Input: part model. Units: mm. Frame: model coordinates. Coordinates: 2 decimals unless noted, no trailing zeros. Write each loop counter-clockwise with the first axis right and the second up, starting at its lowest first coordinate (ties: lowest second). Pieces come first, ordered by that corner, then holes. Notation, with made-up numbers: (47.5, 51.5) -> (106.5, 51.5) arc R7 ccw to (106.5, 63.5) -> close; hole circle Ø5 at (20.25, 31.5). An arc over 180 degrees is marked (long way). Use one line per item in the form item = value. Start each with the question number.
(1) Cut plane C-C on y = 14.5. Return the cut outline in (x, z).
(2) Cut plane B-B on z = 1056. Return the cut outline in (x, y), plus the area to 3 significant figures.
(3) Cut plane A-A on x = -239. Return the cut outline in (y, z).
(4) Ray query, line 1 along Z through (x, y) = (171.5, -68). Return the intervals inside material, ascending.
(5) Pull-direction query (Z, two-part tool) for faces 1 (the face through (-6, 3, 20)), 2 (the face through (-6, 3, 1220)), 3 (the face through (-6, 3, 900)), 4 (the face through (-35, -200, 607)); classes: released by +Z, released by -Z, zero draft, split by the parting line, or undercut.
```python
from build123d import *

# Parameters (mm, degrees)
F4_W      = 900
F4_H      = 400
F6_DEPTH  = 1220
F7_DEPTH  = 280
F11_DEPTH = 280
F12_DEPTH = 280
F13_DEPTH = 280


with BuildPart() as f6:
    # F4 (on Top) → F6 (new body)
    with BuildSketch(Plane.XY):
        Rectangle(F4_W, F4_H)
    extrude(amount=F6_DEPTH)

    # F5 (on offset) → F7 (cut)
    with BuildSketch(Plane.XY.offset(300)):
        Polygon((-430, 198), (-448, 198), (-448, 180), (-450, 180), (-450, -180), (-448, -180), (-448, -198), (-430, -198), (-430, -200), (430, -200), (430, -198), (448, -198), (448, -180), (450, -180), (450, 180), (448, 180), (448, 198), (430, 198), (430, 200), (-430, 200), align=None)
    extrude(amount=-F7_DEPTH, mode=Mode.SUBTRACT)

    # F8 (on offset) → F11 (cut)
    with BuildSketch(Plane.XY.offset(600)):
        Polygon((-430, 198), (-448, 198), (-448, 180), (-450, 180), (-450, -180), (-448, -180), (-448, -198), (-430, -198), (-430, -200), (430, -200), (430, -198), (448, -198), (448, -180), (450, -180), (450, 180), (448, 180), (448, 198), (430, 198), (430, 200), (-430, 200), align=None)
    extrude(amount=-F11_DEPTH, mode=Mode.SUBTRACT)

    # F9 (on offset) → F12 (cut)
    with BuildSketch(Plane.XY.offset(900)):
        Polygon((-430, 198), (-448, 198), (-448, 180), (-450, 180), (-450, -180), (-448, -180), (-448, -198), (-430, -198), (-430, -200), (430, -200), (430, -198), (448, -198), (448, -180), (450, -180), (450, 180), (448, 180), (448, 198), (430, 198), (430, 200), (-430, 200), align=None)
    extrude(amount=-F12_DEPTH, mode=Mode.SUBTRACT)

    # F10 (on offset) → F13 (cut)
    with BuildSketch(Plane.XY.offset(1200)):
        Polygon((-430, 198), (-448, 198), (-448, 180), (-450, 180), (-450, -180), (-448, -180), (-448, -198), (-430, -198), (-430, -200), (430, -200), (430, -198), (448, -198), (448, -180), (450, -180), (450, 180), (448, 180), (448, 198), (430, 198), (430, 200), (-430, 200), align=None)
    extrude(amount=-F13_DEPTH, mode=Mode.SUBTRACT)


solid = f6.part
```
Values:
q1.outline = (-450, 0) -> (450, 0) -> (450, 20) -> (-450, 20) -> close; (-450, 300) -> (450, 300) -> (450, 320) -> (-450, 320) -> close; (-450, 600) -> (450, 600) -> (450, 620) -> (-450, 620) -> close; (-450, 900) -> (450, 900) -> (450, 920) -> (-450, 920) -> close; (-450, 1200) -> (450, 1200) -> (450, 1220) -> (-450, 1220) -> close
q2.outline = (-450, -200) -> (-430, -200) -> (-430, -198) -> (-448, -198) -> (-448, -180) -> (-450, -180) -> close; (-450, 180) -> (-448, 180) -> (-448, 198) -> (-430, 198) -> (-430, 200) -> (-450, 200) -> close; (430, -200) -> (450, -200) -> (450, -180) -> (448, -180) -> (448, -198) -> (430, -198) -> close; (430, 198) -> (448, 198) -> (448, 180) -> (450, 180) -> (450, 200) -> (430, 200) -> close
q2.area = 304 mm2
q3.outline = (-200, 0) -> (200, 0) -> (200, 20) -> (-200, 20) -> close; (-200, 300) -> (200, 300) -> (200, 320) -> (-200, 320) -> close; (-200, 600) -> (200, 600) -> (200, 620) -> (-200, 620) -> close; (-200, 900) -> (200, 900) -> (200, 920) -> (-200, 920) -> close; (-200, 1200) -> (200, 1200) -> (200, 1220) -> (-200, 1220) -> close
q4.line_1 = 0 to 20, 300 to 320, 600 to 620, 900 to 920, 1200 to 1220
q5.face_1 = undercut
q5.face_2 = released by +Z
q5.face_3 = undercut
q5.face_4 = zero draft
